Geometry: final body of the model. Coordinates: model frame, mm. A direction names the side the tool comes from. Round coordinates to 2 decimals unless told otherwise and drop trailing zeros. Loops run counter-clockwise (first coordinate to the right, second up) from the corner with the lowest first, then second, coordinate; pieces in that order, holes last. Notation, with made-up numbers: (3.25, 73) - (15.25, 73) arc R20 ccw to (15.25, 97) - close; hole circle Ø10 at (27, 81). An arc over 180 degrees is marked (long way). Return JSON: item names as keys, results as strings. Group by question number.
1. Section C-C on x = 19.5. Return loops of the section in (y, z).
2. Section B-B on z = 0. Return loops of the section in (x, y).
3. Draft query along X for faces 1 (the face through (11, 0, -25)), 2 (the face through (-11.49, 14.79, 27.712)), 3 (the face through (0, 20, -28)). Return one class per face: +X half, -X half, draft (parallel to the pull), parting line (faces both ways), or undercut.
4. Section A-A on x = 0. Return loops of the section in (y, z).
5. Material intervals for probe 1 along Y at (x, z) = (-29, 0); probe 2 along X at (y, z) = (4.5, 6); probe 3 along X at (y, z) = (6, 20.5), sorted ascending.
6. First-contact query: pin 1 Ø1 at (y, z) = (11.5, 15.5) entering from -X; pin 2 Ø6 at (y, z) = (3, 9) entering from -X; pin 3 Ø3 at (y, z) = (11, -21.5) entering from +X; pin 4 Ø2.5 at (y, z) = (3, 0) entering from -X. Flat tips, straight axial feed; report the tip coordinate or a pass-through.
7. Section D-D on z = -20. Return loops of the section in (x, y).
8. Set-up query: faces 4 (the face through (-28.5, 1.536, 0.325)), 5 (the face through (0, 10, -28)). Return all of +Z, -Z, +X, -X, +Y, -Y with unobstructed straight access to the full face (end or side cutting, diameter ignored); none if empty.
from build123d import *

# Parameters (mm, degrees)
SKETCH2_R               = 30
SKETCH2_R_2             = 27
BOSS_EXTRUDE1_DEPTH     = 30
SKETCH3_W               = 25
SKETCH3_H               = 10
CUT_EXTRUDE3_DEPTH      = 50
CUT_EXTRUDE4_DEPTH      = 52.961524227
CUT_EXTRUDE4_DEPTH_BACK = 52.961524227
SKETCH6_R               = 1.5


with BuildPart() as part:
    # Sketch2 → Boss-Extrude1 (new body)
    with BuildSketch(Plane(origin=(0, 0, 0), x_dir=(1, 0, 0), z_dir=(0, 1, 0))):
        with Locations(Location((0, 0, 0), (0, 0, 270))):
            Circle(SKETCH2_R)
        with Locations(Location((0, 0, 0), (0, 0, 270))):
            Circle(SKETCH2_R_2, mode=Mode.SUBTRACT)
    extrude(amount=BOSS_EXTRUDE1_DEPTH)

    # Sketch3 → Cut-Extrude3 (cut)
    with BuildSketch(Plane.XY):
        with Locations((0, 15)):
            Rectangle(SKETCH3_W, SKETCH3_H)
    extrude(amount=-CUT_EXTRUDE3_DEPTH, mode=Mode.SUBTRACT)

    # Sketch6 → Cut-Extrude4 (cut, two sides: drawn at the far end of the back side and taken through both)
    with BuildSketch(Plane(origin=(0, 0, 0), x_dir=(0, 0, -1), z_dir=(1, 0, 0)).offset(-CUT_EXTRUDE4_DEPTH_BACK)):
        with Locations((0, 3)):
            Circle(SKETCH6_R)
    extrude(amount=CUT_EXTRUDE4_DEPTH + CUT_EXTRUDE4_DEPTH_BACK, mode=Mode.SUBTRACT)


solid = part.part
Taken from the geometry:
{
 "1": {"outline": "(0, -22.8) - (30, -22.8) - (30, -18.67) - (0, -18.67) - close; (0, 18.67) - (30, 18.67) - (30, 22.8) - (0, 22.8) - close"},
 "2": {"outline": "(-30, 0) - (-27, 0) - (-27, 1.5) - (-30, 1.5) - close; (-30, 4.5) - (-27, 4.5) - (-27, 30) - (-30, 30) - close; (27, 0) - (30, 0) - (30, 1.5) - (27, 1.5) - close; (27, 4.5) - (30, 4.5) - (30, 30) - (27, 30) - close"},
 "3": {"face 1": "draft", "face 2": "parting line", "face 3": "undercut"},
 "4": {"outline": "(0, -30) - (10, -30) - (10, -27) - (0, -27) - close; (0, 27) - (30, 27) - (30, 30) - (0, 30) - close; (20, -30) - (30, -30) - (30, -27) - (20, -27) - close"},
 "5": {"probe 1": "0 to 1.5, 4.5 to 30", "probe 2": "-29.39 to -26.32, 26.32 to 29.39", "probe 3": "-21.9 to -17.57, 17.57 to 21.9"},
 "6": {"pin 1": "x = -25.98", "pin 2": "x = -29.39", "pin 3": "x = 22.36", "pin 4": "through"},
 "7": {"outline": "(-22.36, 0) - (-18.14, 0) - (-18.14, 30) - (-22.36, 30) - close; (18.14, 0) - (22.36, 0) - (22.36, 30) - (18.14, 30) - close"},
 "8": {"face 4": "+X, -X", "face 5": "-Z"}
}
